```python
from build123d import *

# Parameters (mm, degrees)
F0_W     = 21
F0_H     = 42
F1_DEPTH = 12
F2_D     = 2.8
F3_W     = 2
F3_H     = 6.526026
F4_DEPTH = 20
F6_W     = 40
F6_H     = 10
F7_DEPTH = 1


with BuildPart() as f1:
    # F0 (on Top) → F1 (new body)
    with BuildSketch(Plane.XY):
        with Locations((10.5, 0)):
            Rectangle(F0_W, F0_H)
    extrude(amount=-F1_DEPTH)

    # F2 (through all)
    with Locations(Plane.XY):
        with Locations((15.75, 15.75), (15.75, -15.75)):
            Hole(F2_D / 2)

    # F3 (on face) → F4 (cut)
    with BuildSketch(Plane(origin=(0, 0, 0), x_dir=(0, -1, 0), z_dir=(-1, 0, 0))):
        Polygon((-20, 0), (-20, -3.214286), (20, -11.785714), (20, 0), align=None)
        Polygon((11.454786, -12), (-19, -5.473974), (-19, -12), align=None)
        with Locations((-20, -8.736987)):
            Rectangle(F3_W, F3_H)
    extrude(amount=-F4_DEPTH, mode=Mode.SUBTRACT)

    # F5: F1 across face


with BuildPart() as f1_1:
    add(f1.part)
    add(f1.part.mirror(Plane(origin=(0, 0.027427, -7.493387), x_dir=(0, -1, 0), z_dir=(-1, 0, 0))))

    # F6 (on face) → F7 (cut)
    with BuildSketch(Plane.XZ.offset(21)):
        with Locations((0, -6)):
            Rectangle(F6_W, F6_H)
    extrude(amount=-F7_DEPTH, mode=Mode.SUBTRACT)


solid = f1_1.part
```
Can you work these out from the model? Positions are in its coordinate system, mm. A direction names the side the tool comes from. Round coordinates to 2 decimals unless told otherwise and drop trailing zeros. Loops run counter-clockwise (first coordinate to the right, second up) from the corner with the lowest first, then second, coordinate; pieces in that order, holes last. Notation, with made-up numbers: M -19.5,79.5 L 34.5,79.5 A18 ccw 34.5,108.5 Z; hole C 40.5,1.5 d1. An arc over 180 degrees is marked long. Answer as a JSON object with one key per item and string values. Group by question number.
Q1. Imagine slicing it at C-C, the plane z = -8. Please give me the cut outline in (x, y).
Q2. Imagine slicing it at A-A, the plane x = 10.5. Please give me the cut outline in (y, z), then the cut area to 3 significant figures.
Q3. On a 3-axis mill with a long thin cutter (end or side, diameter ignored), from which of +Z, -Z, +X, -X, +Y, -Y can I reach the whole of each face in a straight line? I mean faces 1 (the flat face through (0, 20, -2)), 2 (the flat face through (-20, 9, -9)), 3 (the flat face through (-0.3, -20.5, -1)). Say none if no direction works.
Q4. Will these pins go through, and if not, where does the flat tip stop? pin 1 (6 mm diameter, centred on x = -7, y = -6, fed in from -Z); pin 2 (3 mm diameter, centred on x = 15.75, y = 15.75, fed in from +Z); pin 3 (6 mm diameter, centred on x = 5.5, y = 7, fed in from -Z); pin 4 (2.5 mm diameter, centred on x = -15.75, y = -15.75, fed in from +Z).
Q5. Please list where these lines run through material, in increasing order: L1, parallel to X at y = 15.75, z = -5.65; L2, parallel to X at y = 18, z = -8.5; L3, parallel to Y at x = -14, z = -2.5.
Q6. Imagine slicing it at B-B, the plane y = -15.75. Please give me the cut outline in (x, z) (3 decimals), then the cut area to 3 significant figures.
Q7. We'd pull the mould along X, two halves only. Please class faces 4 (the flat face through (0, 21, -3)), 5 (the flat face through (21, 0, -6)), 6 (the cylindrical face through (16.78, 16.7, -5.17)): +X half, -X half, draft (parallel to the pull), parting line (faces both ways), or undercut.
Q8. Imagine slicing it at D-D, the plane x = 15.75. Please give me the cut outline in (y, z) (3 decimals), then the cut area to 3 significant figures.
Findings:
{
 "1": {"outline": "M -21,-21 L -20,-21 L -20,-2.33 L 20,-2.33 L 20,-21 L 21,-21 L 21,21 L 20,21 L 20,7.21 L -20,7.21 L -20,21 L -21,21 Z"},
 "2": {"outline": "M -21,-12 L -11.45,-12 L 19,-5.47 L 21,-5.47 L 21,0 L 20,0 L 20,-3.21 L -20,-11.79 L -20,-11 L -21,-11 Z; M -21,-1 L -20,-1 L -20,0 L -21,0 Z", "area": "81.6 mm2"},
 "3": {"face 1": "+Z", "face 2": "-Z, +Y", "face 3": "-Y"},
 "4": {"pin 1": "stops at z = -11.47", "pin 2": "stops at z = -3.8", "pin 3": "stops at z = -8.69", "pin 4": "passes through"},
 "5": {"L1": "x = -21 to -17.15, -14.35 to 14.35, 17.15 to 21", "L2": "x = -21 to -20, 20 to 21", "L3": "y = 20 to 21"},
 "6": {"outline": "M -21,-12 L -17.15,-12 L -17.15,-10.875 L -20,-10.875 L -20,0 L -21,0 Z; M -14.35,-12 L 14.35,-12 L 14.35,-10.875 L -14.35,-10.875 Z; M 17.15,-12 L 21,-12 L 21,0 L 20,0 L 20,-10.875 L 17.15,-10.875 Z", "area": "62.7 mm2"},
 "7": {"face 4": "draft", "face 5": "+X half", "face 6": "undercut"},
 "8": {"outline": "M -21,-12 L -17.15,-12 L -17.15,-11.175 L -20,-11.786 L -20,-11 L -21,-11 Z; M -21,-1 L -20,-1 L -20,0 L -21,0 Z; M -14.35,-12 L -11.455,-12 L 14.35,-6.47 L 14.35,-4.425 L -14.35,-10.575 Z; M 17.15,-5.87 L 19,-5.474 L 21,-5.474 L 21,0 L 20,0 L 20,-3.214 L 17.15,-3.825 Z", "area": "72.7 mm2"}
}
